```python
from build123d import *

# Parameters (mm, degrees)
SKETCH_W         = 34
SKETCH_H         = 75
PAD_DEPTH        = 5
SKETCH001_W      = 34
SKETCH001_H      = 20
PAD001_DEPTH     = 15
SKETCH002_W      = 27
SKETCH002_H      = 10.5
POCKET_DEPTH     = 10
HOLE_D           = 4.8
HOLE_DEPTH       = 25
HOLE_CBORE_D     = 8.25
HOLE_CBORE_DEPTH = 4
SKETCH004_R      = 2
SKETCH004_W      = 2
SKETCH004_H      = 8
POCKET001_DEPTH  = 5
CHAMFER_SIZE     = 5


with BuildPart() as part:
    # Sketch → Pad (new body)
    with BuildSketch(Plane.XY):
        Rectangle(SKETCH_W, SKETCH_H)
    extrude(amount=PAD_DEPTH)

    # Sketch001 (on Face6 of Pad) → Pad001 (join)
    with BuildSketch(Plane.XY.offset(5)):
        with Locations((0, -27.5)):
            Rectangle(SKETCH001_W, SKETCH001_H)
    extrude(amount=PAD001_DEPTH)

    # Sketch002 (on Face10 of Pad001) → Pocket (cut)
    with BuildSketch(Plane.XY.offset(20)):
        with Locations((0, -27.5)):
            Rectangle(SKETCH002_W, SKETCH002_H)
    extrude(amount=-POCKET_DEPTH, mode=Mode.SUBTRACT)

    # Hole
    with Locations(Plane(origin=(0, 0, 0), x_dir=(1, 0, 0), z_dir=(0, 0, -1))):
        with Locations((-6.5, 27.5), (6.5, 27.5)):
            CounterBoreHole(HOLE_D / 2, HOLE_CBORE_D / 2, HOLE_CBORE_DEPTH, depth=HOLE_DEPTH)

    # Sketch004 (on Face5 of Hole) → Pocket001 (cut)
    with BuildSketch(Plane.XY.offset(5)):
        with Locations((0, 30)):
            Circle(SKETCH004_R)
        with Locations((0, -2.5)):
            Circle(SKETCH004_R)
        with Locations((-13, 30)):
            Rectangle(SKETCH004_W, SKETCH004_H)
        with Locations((13, 30)):
            Rectangle(SKETCH004_W, SKETCH004_H)
        with Locations((-13, -2.5)):
            Rectangle(SKETCH004_W, SKETCH004_H)
        with Locations((13, -2.5)):
            Rectangle(SKETCH004_W, SKETCH004_H)
    extrude(amount=-POCKET001_DEPTH, mode=Mode.SUBTRACT)

    # Chamfer
    chamfer_edges = [part.edges().sort_by_distance(p)[0] for p in [
        (0, -17.5, 5),
    ]]
    chamfer(chamfer_edges, length=CHAMFER_SIZE)


solid = part.part
```
Read the model definition and answer for the solid it produces. Units are mm, in the model's axes. A direction names the side the tool comes from. Give positions to 0.01 mm unless a question says otherwise; leave off trailing zeros. Order: outer loops, then holes, each group sorted by start corner. A loop starts at its lowest first (then second) coordinate and runs counter-clockwise, first axis right, second up. Notation, with made-up numbers: (61, 51.5) -> (73, 51.5) arc R38 cw to (73, 90.5) -> close; hole circle Ø8 at (69, -13.5). An arc over 180 degrees is marked (long way). Write item = value, one per line.
1. Straight lines are drawn through the part: line 1 along X through (y, z) = (-27.5, 1.75) (3 decimals); line 2 along Y through (x, z) = (6.5, 0.9) (3 decimals); line 3 along Y through (x, z) = (-9, 19). For each, find the intervals that lie inside material, in ascending order.
Numbers:
line_1 = -17 to -10.625, -2.375 to 2.375, 10.625 to 17
line_2 = -37.5 to -31.625, -23.375 to 37.5
line_3 = -37.5 to -32.75, -22.25 to -17.5
2. A cutting plane is placed at A-A, the plane y = -5.5. Write down the section's boundary in (x, z), and give its area (3 significant figures).
Numbers:
outline = (-17, 0) -> (-14, 0) -> (-14, 5) -> (-17, 5) -> close; (-12, 0) -> (12, 0) -> (12, 5) -> (-12, 5) -> close; (14, 0) -> (17, 0) -> (17, 5) -> (14, 5) -> close
area = 150 mm²
3. The mould has two halves that part along X. Classify faces 4 (the face through (17, -17, 5)), 5 (the face through (-13, -6.5, 3)), 6 (the face through (-17, -17, 5)), 7 (the face through (-0.434, -4.452, 2.535)): +X half, -X half, draft (parallel to the pull), parting line (faces both ways), or undercut.
Numbers:
face_4 = +X half
face_5 = undercut
face_6 = -X half
face_7 = undercut
4. A cutting plane is placed at D-D, the plane y = -27.5. Write down the section's boundary in (x, z) (3 decimals), and give its area (3 significant figures).
Numbers:
outline = (-17, 0) -> (-10.625, 0) -> (-10.625, 4) -> (-8.9, 4) -> (-8.9, 10) -> (-13.5, 10) -> (-13.5, 20) -> (-17, 20) -> close; (-4.1, 4) -> (-2.375, 4) -> (-2.375, 0) -> (2.375, 0) -> (2.375, 4) -> (4.1, 4) -> (4.1, 10) -> (-4.1, 10) -> close; (8.9, 4) -> (10.625, 4) -> (10.625, 0) -> (17, 0) -> (17, 20) -> (13.5, 20) -> (13.5, 10) -> (8.9, 10) -> close
area = 286 mm²
5. A cutting plane is placed at C-C, the plane z = 6. Write down the section's boundary in (x, y).
Numbers:
outline = (-17, -37.5) -> (17, -37.5) -> (17, -13.5) -> (-17, -13.5) -> close; hole circle Ø4.8 at (-6.5, -27.5); hole circle Ø4.8 at (6.5, -27.5)
6. Given pin 1 (5 mm diameter, centred on x = -0.5, y = -26, fed in from +Z); pin 2 (10 mm diameter, centred on y = -11.5, z = 16.5, fed in from -X); pin 3 (11 mm diameter, centred on x = 1, z = 17.5, fed in from +Y), each flat-ended and moving along its own axis, determine where each tip first touches the part or whether it passes through.
Numbers:
pin_1 = 10
pin_2 = through
pin_3 = -17.5
7. For faces 1 (the face through (13, 1.5, 3)), 2 (the face through (0, -17.5, 15)), 3 (the face through (-7.04, -31.59, 1.97)), determine the directions among +Z, -Z, +X, -X, +Y, -Y from which every point of the face is accessible in a straight line to the end or side of a thin tool.
Numbers:
face_1 = +Z, -Z
face_2 = +Z, +X, -X, +Y
face_3 = -Z
8. A cutting plane is placed at B-B, the plane x = 6.5. Write down the section's boundary in (y, z) (3 decimals), and give its area (3 significant figures).
Numbers:
outline = (-37.5, 0) -> (-31.625, 0) -> (-31.625, 4) -> (-29.9, 4) -> (-29.9, 10) -> (-32.75, 10) -> (-32.75, 20) -> (-37.5, 20) -> close; (-25.1, 4) -> (-23.375, 4) -> (-23.375, 0) -> (37.5, 0) -> (37.5, 5) -> (-12.5, 5) -> (-17.5, 10) -> (-17.5, 20) -> (-22.25, 20) -> (-22.25, 10) -> (-25.1, 10) -> close
area = 521 mm²
